from build123d import *

# Parameters (mm, degrees)
F0_R     = 54.489466
F1_DEPTH = 64.704746
F2_R     = 39.061094
F3_DEPTH = 64.705746
F5_DEPTH = 9.179119
F7_DEPTH = 37.812758
F9_DEPTH = 61.671157


with BuildPart() as f1:
    # F0 (on Top) → F1 (new body)
    with BuildSketch(Plane.XY):
        with Locations((0, 42.404458)):
            Circle(F0_R)
    extrude(amount=F1_DEPTH)

    # F2 (on face) → F3 (cut, through all)
    with BuildSketch(Plane.XY.offset(64.704746)):
        with Locations((0, 42.404458)):
            Circle(F2_R)
    extrude(amount=-F3_DEPTH, mode=Mode.SUBTRACT)

    # F4 (on Top) → F5 (join)
    with BuildSketch(Plane.XY):
        with BuildLine():
            ThreePointArc((38.466547, 5.618665), (-2.008565, -13.031675), (-41.539069, 7.545232))
            Line((-41.539069, 7.545232), (-41.539069, -75.912714))
            Line((-41.539069, -75.912714), (38.466547, -75.912714))
            Line((38.466547, -75.912714), (38.466547, 5.618665))
        make_face()
    extrude(amount=F5_DEPTH)

    # F6 (on face) → F7 (join)
    with BuildSketch(Plane.XY.offset(9.179119)):
        with BuildLine():
            ThreePointArc((7.180691, -12.414793), (-0.887242, -13.282551), (-8.9518, -12.38397))
            Line((-8.9518, -12.38397), (-8.9518, -50.31085))
            Line((-8.9518, -50.31085), (7.180691, -50.31085))
            Line((7.180691, -50.31085), (7.180691, -12.414793))
        make_face()
    extrude(amount=F7_DEPTH)

    # F8 (on face) → F9 (cut, through all)
    with BuildSketch(Plane.YZ.offset(7.180691)):
        Polygon((-50.31085, 9.179119), (-12.414793, 46.991877), (-50.31085, 46.991877), align=None)
    extrude(amount=-F9_DEPTH, mode=Mode.SUBTRACT)


solid = f1.part
Source: CAD feature listing. Evaluate the final solid. Frame: model axes, mm. A direction names the side the tool comes from. Give positions to 0.01 mm unless a question says otherwise; leave off trailing zeros. Order: outer loops, then holes, each group sorted by start corner. A loop starts at its lowest first (then second) coordinate and runs counter-clockwise, first axis right, second up. Notation, with made-up numbers: (65, 26) -> (85, 26) arc R25 cw to (85, 61) -> close; hole circle Ø4 at (12.25, -28). An arc over 180 degrees is marked (long way). Write item = value, one per line.
Item 1: Section query C-C (y = -2). Output: boundary loops of the cut face in (x, z), then the cut area to 3 significant figures.
Check result:
outline = (-41.54, 0) -> (-32.35, 0) -> (-32.35, 9.18) -> (-41.54, 9.18) -> close; (-31.58, 0) -> (38.47, 0) -> (38.47, 9.18) -> (31.58, 9.18) -> (31.58, 64.7) -> (-31.58, 64.7) -> close
area = 4,230 mm²
Item 2: Mould query, pull axis Y, two halves, no side actions, for faces 1 (the face through (-2, -75.913, 5)), 2 (the face through (-8.47, -12.46, 4.53)), 3 (the face through (-1, -8, 0)), 4 (the face through (-31, 18.64, 32.81)). Classes: +Y half, -Y half, draft (parallel to the pull), parting line (faces both ways), or undercut.
Check result:
face_1 = -Y half
face_2 = undercut
face_3 = draft
face_4 = undercut
Item 3: Section query B-B (x = -21). Output: boundary loops of the cut face in (y, z).
Check result:
outline = (-75.91, 0) -> (-8.84, 0) -> (-8.84, 9.18) -> (-75.91, 9.18) -> close; (-7.88, 0) -> (9.47, 0) -> (9.47, 64.7) -> (-7.88, 64.7) -> close; (75.34, 0) -> (92.68, 0) -> (92.68, 64.7) -> (75.34, 64.7) -> close
Item 4: Section query A-A (z = 17.5). Output: boundary loops of the cut face in (x, y).
Check result:
outline = circle Ø108.98 at (0, 42.4); (-8.95, -41.97) -> (7.18, -41.97) -> (7.18, -12.41) arc R37.28 cw to (-8.95, -12.38) -> close; hole circle Ø78.12 at (0, 42.4)
Item 5: Contact query for flat-ended pins moving along their axis: pin 1 (2 mm diameter, centred on x = -19.5, z = 10.5, fed in from +Y); pin 2 (4 mm diameter, centred on x = 7, z = 39, fed in from -Y); pin 3 (4.5 mm diameter, centred on y = -43.5, z = 3, fed in from +X). Output: stop coordinate, or through.
Check result:
pin_1 = 93.66
pin_2 = -22.43
pin_3 = 38.47
Item 6: Set-up query: faces 5 (the face through (38.467, -37, 5)), 6 (the face through (-11, -43, 9.179)), 7 (the face through (-0.773, -13.283, 27.821)), 8 (the face through (-8.952, -27, 24)). Return all of +Z, -Z, +X, -X, +Y, -Y with unobstructed straight access to the full face (end or side cutting, diameter ignored); none if empty.
Check result:
face_5 = +Z, -Z, +X, -Y
face_6 = +Z, -Y
face_7 = +Z
face_8 = +Z, -X, -Y
Item 7: Ray query, probe 1 along Y at (x, z) = (0, 39) (3 decimals); probe 2 along Y at (x, z) = (-2.5, 24.5); probe 3 along X at (y, z) = (-8, 3). Return the intervals inside material, ascending.
Check result:
probe_1 = -20.424 to -13.274, -12.085 to 3.343, 81.466 to 96.894
probe_2 = -34.96 to -13.24, -12.03 to 3.42, 81.39 to 96.84
probe_3 = -41.54 to -22.82, -20.7 to 20.7, 21.24 to 38.47
Item 8: Section query D-D (z = 27). Output: boundary loops of the cut face in (x, y), then the cut area to 3 significant figures.
Check result:
outline = circle Ø108.98 at (0, 42.4); (-8.95, -32.45) -> (7.18, -32.45) -> (7.18, -12.41) arc R37.28 cw to (-8.95, -12.38) -> close; hole circle Ø78.12 at (0, 42.4)
area = 4,850 mm²
